```python
from build123d import *

# Parameters (mm, degrees)
SKETCH_R        = 10.5
PAD_DEPTH       = 17
CHAMFER_SIZE    = 1
CHAMFER001_SIZE = 1


with BuildPart() as part:
    # Sketch → Pad (new body)
    with BuildSketch(Plane.XY):
        Circle(SKETCH_R)
    extrude(amount=PAD_DEPTH)

    # Chamfer
    chamfer_edges = [part.edges().sort_by_distance(p)[0] for p in [
        (-10.5, 0, 17),
    ]]
    chamfer(chamfer_edges, length=CHAMFER_SIZE)

    # Chamfer001
    chamfer001_edges = [part.edges().sort_by_distance(p)[0] for p in [
        (-10.5, 0, 0),
    ]]
    chamfer(chamfer001_edges, length=CHAMFER001_SIZE)


solid = part.part
```
Work out the finished part from the listing and answer in its coordinate system (mm). Round coordinates to 2 decimals unless told otherwise and drop trailing zeros. Write each loop counter-clockwise with the first axis right and the second up, starting at its lowest first coordinate (ties: lowest second). Pieces come first, ordered by that corner, then holes. Notation, with made-up numbers: (64.25, 1.25) - (111.25, 1.25) arc R20 ccw to (111.25, 40.25) - close; hole circle Ø2 at (40.25, -3). An arc over 180 degrees is marked (long way). Return JSON: item names as keys, results as strings. Group by question number.
Q1. Find the intervals of material crossed by L1, parallel to Y at x = 0.25, z = 6.75; L2, parallel to X at y = -8.75, z = 11.5; L3, parallel to X at y = -8.5, z = 6.75, in increasing order.
Q2. The part is cut by section A-A on z = 11.25. Write down the section's boundary in (x, y).
Q3. Each of these flat-tipped pins is pushed along its axis until it touches: pin 1 Ø6 at (x, z) = (5.5, 7) entering from +Y; pin 2 Ø1 at (x, y) = (6, 0.5) entering from -Z; pin 3 Ø1.5 at (y, z) = (6, 6) entering from +X; pin 4 Ø3 at (y, z) = (3.5, 7) entering from -X. Where does it stop, or does it pass through?
Q4. The mould has two halves that part along X. Classify faces 1 (the flat face through (0, 0, 17)), 2 (the cylindrical face through (10, 3.2, 8.4)): released by +X, released by -X, zero draft, split by the parting line, or undercut.
Solved:
{
 "1": {"L1": "-10.5 to 10.5", "L2": "-5.8 to 5.8", "L3": "-6.16 to 6.16"},
 "2": {"outline": "circle Ø21 at (0, 0)"},
 "3": {"pin 1": "y = 10.2", "pin 2": "z = 0", "pin 3": "x = 9.09", "pin 4": "x = -10.31"},
 "4": {"face 1": "zero draft", "face 2": "split by the parting line"}
}
